Work out the finished part from the listing and answer in its coordinate system (mm). Face numbers are marked on the shaded views. A direction names the side the tool comes from. Coordinates: 2 decimals unless noted, no trailing zeros. Order: outer loops, then holes, each group sorted by start corner. A loop starts at its lowest first (then second) coordinate and runs counter-clockwise, first axis right, second up. Notation, with made-up numbers: M 5,25 L 18,25 A25 cw 18,40 Z; hole C 65,78.25 d7. An arc over 180 degrees is marked long. Use a Markdown table: item, result.
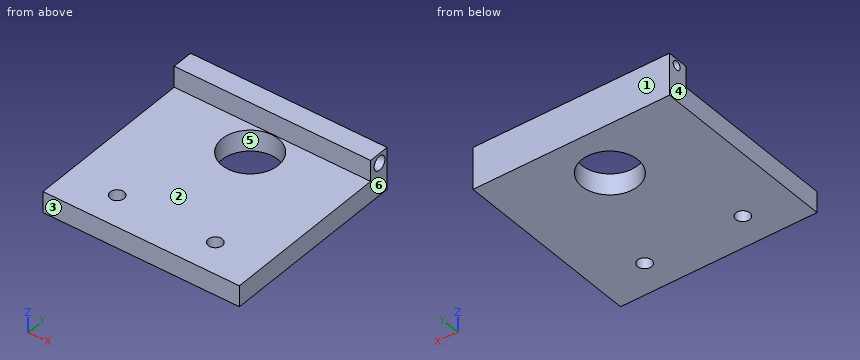
from build123d import *

# Parameters (mm, degrees)
F0_W     = 88.9
F0_H     = 82.55
F0_R     = 12.7
F2_DEPTH = 9.525
F1_W     = 9.525
F1_H     = 19.05
F3_DEPTH = 44.45
F4_R     = 3.175
F5_DEPTH = 25.4
F6_R     = 2.0432827377
F7_DEPTH = 19.05
F8_R     = 3.175
F9_DEPTH = 19.051


with BuildPart() as f2:
    # F0 (on Top) → F2 (new body)
    with BuildSketch(Plane.XY):
        Rectangle(F0_W, F0_H)
        with Locations((0, 22.225)):
            Circle(F0_R, mode=Mode.SUBTRACT)
    extrude(amount=F2_DEPTH)

    # F1 (on Right) → F3 (join, symmetric)
    with BuildSketch(Plane.YZ):
        with Locations((39.9805786431, 9.525)):
            Rectangle(F1_W, F1_H)
    extrude(amount=F3_DEPTH, both=True)

    # F4 (on face) → F5 (cut)
    with BuildSketch(Plane.YZ.offset(44.45)):
        with Locations((40.4250786431, 14.605)):
            Circle(F4_R)
    extrude(amount=-F5_DEPTH, mode=Mode.SUBTRACT)

    # F6 (on face) → F7 (cut)
    with BuildSketch(Plane(origin=(-44.45, 0, 0), x_dir=(0, -1, 0), z_dir=(-1, 0, 0))):
        with Locations((-40.5182726681, 16.0620938987)):
            Circle(F6_R)
    extrude(amount=-F7_DEPTH, mode=Mode.SUBTRACT)

    # F8 (on face) → F9 (cut, through all)
    with BuildSketch(Plane(origin=(0, 0, 0), x_dir=(1, 0, 0), z_dir=(0, 0, -1))):
        with Locations((22.2250018269, 26.67)):
            Circle(F8_R)
        with Locations((-22.225, 26.67)):
            Circle(F8_R)
    extrude(amount=-F9_DEPTH, mode=Mode.SUBTRACT)


solid = f2.part
1. For a pull along X with two mould halves and no side action, classify the marked faces 3, 4, 5 and 6 as +X half, -X half, draft (parallel to the pull), parting line (faces both ways), or undercut.
Answers below:
| item | result |
|---|---|
| face 3 | draft |
| face 4 | -X half |
| face 5 | undercut |
| face 6 | +X half |
2. Section C-C on z = 5.75 is taken. Determine the outline of the cut face in (x, y) (3 decimals), then the cut area to 3 significant figures.
Answers below:
| item | result |
|---|---|
| outline | M -44.45,-41.275 L 44.45,-41.275 L 44.45,44.743 L -44.45,44.743 Z; hole C -22.225,-26.67 d6.35; hole C 0,22.225 d25.4; hole C 22.225,-26.67 d6.35 |
| area | 7,080 mm² |
3. Find the intervals of material crossed by probe 1 along X at (y, z) = (-26.67, 6); probe 2 along X at (y, z) = (22, 8); probe 3 along Y at (x, z) = (0, 5.25) (3 decimals), in increasing order.
Answers below:
| item | result |
|---|---|
| probe 1 | -44.45 to -25.4, -19.05 to 19.05, 25.4 to 44.45 |
| probe 2 | -44.45 to -12.7, 12.7 to 44.45 |
| probe 3 | -41.275 to 9.525, 34.925 to 44.743 |
4. Section A-A on x = 0 is taken. Determine the outline of the cut face in (y, z) (3 decimals), then the cut area to 3 significant figures.
Answers below:
| item | result |
|---|---|
| outline | M -41.275,0 L 9.525,0 L 9.525,9.525 L -41.275,9.525 Z; M 34.925,0 L 44.743,0 L 44.743,19.05 L 35.218,19.05 L 35.218,9.525 L 34.925,9.525 Z |
| area | 668 mm² |
5. Section D-D on x = -34 is taken. Determine the outline of the cut face in (y, z) (3 decimals).
Answers below:
| item | result |
|---|---|
| outline | M -41.275,0 L 44.743,0 L 44.743,19.05 L 35.218,19.05 L 35.218,9.525 L -41.275,9.525 Z; hole C 40.518,16.062 d4.087 |
6. For the marked faces 1 and 2, determine the directions among +Z, -Z, +X, -X, +Y, -Y from which every point of the face is accessible in a straight line to the end or side of a thin tool.
Answers below:
| item | result |
|---|---|
| face 1 | +Z, -Z, +X, -X, +Y |
| face 2 | +Z, +X, -X, -Y |
7. Section B-B on y = -26.67 is taken. Determine the outline of the cut face in (x, z) (3 decimals).
Answers below:
| item | result |
|---|---|
| outline | M -44.45,0 L -25.4,0 L -25.4,9.525 L -44.45,9.525 Z; M -19.05,0 L 19.05,0 L 19.05,9.525 L -19.05,9.525 Z; M 25.4,0 L 44.45,0 L 44.45,9.525 L 25.4,9.525 Z |
8. Flat-ended cylindrical pins translate along their axes: P1, Ø1.9, axis at y = 40.5, z = 16, coming from the +X side; P2, Ø8.5, axis at x = 22.23, y = -26.67, coming from the +Z side (3 decimals); P3, Ø3, axis at x = -18, z = 14, coming from the -Y side. Find the tip coordinate at first contact, or state that the pin passes through.
Answers below:
| item | result |
|---|---|
| P1 | x = 19.05 |
| P2 | z = 9.525 |
| P3 | y = 35.22 |
